The model under review builds one solid part; all positions refer to its coordinate system, in mm. Face numbers are marked on the shaded views. A direction names the side the tool comes from. Round coordinates to 2 decimals unless told otherwise and drop trailing zeros. Order: outer loops, then holes, each group sorted by start corner. A loop starts at its lowest first (then second) coordinate and runs counter-clockwise, first axis right, second up. Notation, with made-up numbers: M -21,-6.5 L 38,-6.5 A15 ccw 38,13.5 Z; hole C 74,12.25 d8. An arc over 180 degrees is marked long. Use a Markdown table: item, result. Add a question column.
1. Consider section B-B on x = 2. State the section outline as (y, z) points.
2. The part is to be moulded in two halves that separate along Z. For the marked faces 1, 2 and 3, say which applies: +Z half, -Z half, draft (parallel to the pull), parting line (faces both ways), or undercut.
3. Consider section A-A on x = 8. State the section outline as (y, z) points.
4. Insertion check: P1, Ø12, axis at x = 15.5, z = 16.5, coming from the -Y side; P2, Ø6, axis at y = 5, z = 11.5, coming from the +X side; P3, Ø5, axis at x = -2, y = -3, coming from the +Z side; P4, Ø8, axis at x = -16, z = 15.5, coming from the -Y side. Each pin has a flat end and moves straight along its axis. Give the tip position at first contact, or say it passes through.
5. Consider section D-D on z = 19.25. State the section outline as (x, y) points, then the cut area to 3 significant figures.
6. For the marked faces 4, 5, 6, 7 and 8, list the 3-axis set-ups (+Z, -Z, +X, -X, +Y, -Y) from which the entire face can be reached by the end or side of a thin tool; tool diameter is ignored.
7. To check wall thickness, follow probe 1 along Z at (x, y) = (-18, 2.25); probe 2 along Y at (x, z) = (-7, 7); probe 3 along X at (y, z) = (-0.25, 9.5). State the ranges of each line that lie inside material, in increasing order.
8. Consider section C-C on y = -3.75. State the section outline as (x, z) points, then the cut area to 3 significant figures.
from build123d import *

# Parameters (mm, degrees)
F4_DEPTH = 3
F5_DEPTH = 7.5
F3_W     = 4.5
F3_H     = 2.25
F6_DEPTH = 2
F7_R     = 3


with BuildPart() as f4:
    # F3 (on Front) → F4 (new body, symmetric)
    with BuildSketch(Plane.XZ):
        Polygon((-7.5, 18.6698729811), (-7.5, 1), (7.5, 1), (7.5, 18.6698729811), (15, 23), (15, 25), (10.5, 25), (-10.5, 25), (-15, 25), (-15, 23), align=None)
    extrude(amount=F4_DEPTH, both=True)

    # F3 (on Front) → F5 (join, symmetric)
    with BuildSketch(Plane.XZ):
        Polygon((-22.5, 1), (-22.5, 0), (22.5, 0), (22.5, 1), (7.5, 1), (-7.5, 1), align=None)
    extrude(amount=F5_DEPTH, both=True)

    # F3 (on Front) → F6 (join, symmetric)
    with BuildSketch(Plane.XZ):
        with Locations((12.75, 26.125)):
            Rectangle(F3_W, F3_H)
        with Locations((-12.75, 26.125)):
            Rectangle(F3_W, F3_H)
    extrude(amount=F6_DEPTH, both=True)

    # F7
    f7_edges = [f4.edges().sort_by_distance(p)[0] for p in [
        (22.5, -7.5, 0.5),
        (22.5, 7.5, 0.5),
        (-22.5, 7.5, 0.5),
        (-22.5, -7.5, 0.5),
    ]]
    fillet(f7_edges, radius=F7_R)


solid = f4.part
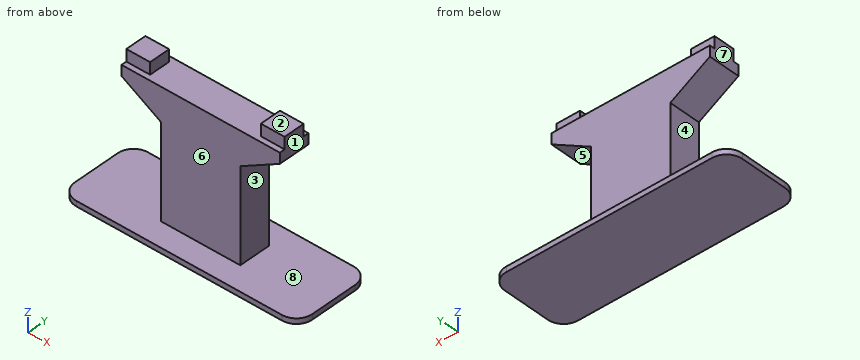
Answer block:
| question | item | result |
|---|---|---|
| 1 | outline | M -7.5,0 L 7.5,0 L 7.5,1 L 3,1 L 3,25 L -3,25 L -3,1 L -7.5,1 Z |
| 2 | face 1 | draft |
| 2 | face 2 | +Z half |
| 2 | face 3 | undercut |
| 3 | outline | M -7.5,0 L 7.5,0 L 7.5,1 L -7.5,1 Z; M -3,18.96 L 3,18.96 L 3,25 L -3,25 Z |
| 4 | P1 | y = -3 |
| 4 | P2 | x = 7.5 |
| 4 | P3 | z = 25 |
| 4 | P4 | through |
| 5 | outline | M -8.5,-3 L 8.5,-3 L 8.5,3 L -8.5,3 Z |
| 5 | area | 102 mm^2 |
| 6 | face 4 | -X, +Y, -Y |
| 6 | face 5 | +X, +Y, -Y |
| 6 | face 6 | +Z, +X, -X, -Y |
| 6 | face 7 | +Z, -X, +Y, -Y |
| 6 | face 8 | none |
| 7 | probe 1 | 0 to 1 |
| 7 | probe 2 | -3 to 3 |
| 7 | probe 3 | -7.5 to 7.5 |
| 8 | outline | M -22.5,0 L 22.5,0 L 22.5,1 L -22.5,1 Z |
| 8 | area | 45.0 mm^2 |
